Design review of the part built by this model. Coordinates are the model's own, in mm. Coordinates: 2 decimals unless noted, no trailing zeros. Loops run counter-clockwise (first coordinate to the right, second up) from the corner with the lowest first, then second, coordinate; pieces in that order, holes last. Notation, with made-up numbers: M 42.5,-5 L 87.5,-5 A20 cw 87.5,6 Z; hole C -2,25.5 d9. An arc over 180 degrees is marked long. Put each result on its own line as item: value. Start each with the question number.
(1) Take a section at A-A, the plane x = -80.5. Give the boundary of the cut face in (y, z).
(2) Take a section at D-D, the plane x = -41. Give the boundary of the cut face in (y, z).
(3) Clearance check with flat-ended pins moving along their axes: pin 1 (1.5 mm diameter, centred on x = -9.5, y = -12, fed in from -Z); pin 2 (8 mm diameter, centred on y = -18.5, z = 32, fed in from +X); pin 3 (10 mm diameter, centred on y = -20.5, z = 5, fed in from +X); pin 4 (1.5 mm diameter, centred on x = -56, z = 53, fed in from +Y). State where each tip first meets the part, or that it passes through.
(4) Take a section at C-C, the plane y = -3. Give the boundary of the cut face in (x, z), then the cut area to 3 significant figures.
(5) The part is to be moulded in two halves that separate along Z. For faces 1 (the cylindrical face through (-84.688, -13.242, -53.617)), 2 (the cylindrical face through (15.94, -13.24, 42.22)), say which applies: +Z half, -Z half, draft (parallel to the pull), parting line (faces both ways), or undercut.
(6) Take a section at B-B, the plane z = 35.5. Give the boundary of the cut face in (x, y), then the cut area to 3 significant figures.
(7) For probe 1 along Z at (x, y) = (-55.5, -5); probe 2 along X at (y, z) = (-14, 12); probe 3 along Z at (x, y) = (-31, -21.75), list the stretches that pass through material, from the lowest coordinate up. Write a range as [from, to].
```python
from build123d import *

# Parameters (mm, degrees)
F0_W      = 54.628875
F0_H      = 26.859861
F1_DEPTH  = 61.468
F1_FACE_W = 54.628876
F1_FACE_H = 26.85986


with BuildPart() as f1:
    # F0 (on Top) → F1 (new body)
    with BuildSketch(Plane.XY):
        with Locations((-27.314438, -13.42993)):
            Rectangle(F0_W, F0_H)
    extrude(amount=F1_DEPTH)

    # F1_face (on face) → F2 (revolve)
    with BuildSketch(Plane(origin=(-27.314438, -13.42993, 61.468), x_dir=(1, 0, 0), z_dir=(0, 0, 1))):
        Rectangle(F1_FACE_W, F1_FACE_H)
    revolve(axis=Axis((-54.628875, -13.42993, 0), (0, 1, 0)))


solid = f1.part
```
Computed values:
1. outline: M -26.86,-78.06 L 0,-78.06 L 0,-55.76 L -26.86,-55.76 Z; M -26.86,55.76 L 0,55.76 L 0,78.06 L -26.86,78.06 Z
2. outline: M -26.86,-81.1 L 0,-81.1 L 0,-59.94 L -26.86,-59.94 Z; M -26.86,0 L 0,0 L 0,81.1 L -26.86,81.1 Z
3. pin 1: stops at z = -69.23
3. pin 2: stops at x = 22.69
3. pin 3: stops at x = 27.61
3. pin 4: passes through
4. outline: C -54.63,0 d164.47; hole M -54.63,0 L -54.63,61.47 A61.47 ccw long 0,28.18 L 0,0 Z
4. area: 12,200 mm^2
5. face 1: undercut
5. face 2: parting line
6. outline: M -128.81,-26.86 L -104.81,-26.86 L -104.81,0 L -128.81,0 Z; M -54.63,-26.86 L 19.55,-26.86 L 19.55,0 L -54.63,0 Z
6. area: 2,640 mm^2
7. probe 1: z = [-82.23, -61.46], [61.46, 82.23]
7. probe 2: x = [-135.98, -114.91], [-54.63, 0], [5.66, 26.73]
7. probe 3: z = [-78.77, -56.74], [0, 78.77]
